from build123d import *

# Parameters (mm, degrees)
SCHIZZO1_W                   = 30
SCHIZZO1_H                   = 12
SCHIZZO1_R                   = 2.5
ESTRUSIONE_ESTRUSIONE1_DEPTH = 7.5
TAGLIO_ESTRUSIONE1_REACH     = 33.5
SCHIZZO3_R                   = 2.5


with BuildPart() as part:
    # Schizzo1 → Estrusione-Estrusione1 (new, symmetric)
    with BuildSketch(Plane.XY):
        Rectangle(SCHIZZO1_W, SCHIZZO1_H)
        Circle(SCHIZZO1_R, mode=Mode.SUBTRACT)
    extrude(amount=ESTRUSIONE_ESTRUSIONE1_DEPTH, both=True)

    # Taglio-Estrusione1: up to this face of the body (flat: up to its plane)
    taglio_estrusione1_end = Plane(part.part.faces().sort_by_distance((-15, 0, 0))[0])
    # Schizzo3 → Taglio-Estrusione1 (cut, up to the picked face)
    with BuildSketch(Plane(origin=(15, 0, 0), x_dir=(0, 0, -1), z_dir=(1, 0, 0)), mode=Mode.PRIVATE) as taglio_estrusione1_sk1:
        Circle(SCHIZZO3_R)
    taglio_estrusione1_tool1 = split(extrude(taglio_estrusione1_sk1.sketch, amount=-TAGLIO_ESTRUSIONE1_REACH, mode=Mode.PRIVATE), bisect_by=taglio_estrusione1_end, keep=Keep.BOTH, mode=Mode.PRIVATE)
    add(taglio_estrusione1_tool1.solids().sort_by(Axis((15, 0, 0), (-1, 0, 0)))[0], mode=Mode.SUBTRACT)


solid = part.part
Part model, mm, in its own coordinate system. Coordinates: 2 decimals unless noted, no trailing zeros. Loops run counter-clockwise (first coordinate to the right, second up) from the corner with the lowest first, then second, coordinate; pieces in that order, holes last. Notation, with made-up numbers: (-26, 4) -> (20, 4) arc R16 cw to (20, 9) -> close; hole circle Ø1 at (-27.75, 28). An arc over 180 degrees is marked (long way). Use a Markdown table: item, result. Add a question column.
Item 1: Band-saw the part on C-C on z = -3. Write the cut outline in (x, y).
Item 2: Flat gauge pin, fed straight in: P1, Ø6.5, axis at x = 0, y = 0, coming from the +Z side. Where does the tip first touch, or does it go through?
Item 3: Band-saw the part on A-A on y = 0. Write the cut outline in (x, z), plus the area to 3 significant figures.
Item 4: Probe probe 1 along Y at (x, z) = (1, 0); probe 2 along Z at (x, y) = (9.25, 0); probe 3 along X at (y, z) = (-0.25, -4). List the from-to ranges inside material, lowest first.
Item 5: Band-saw the part on D-D on x = -1. Write the cut outline in (y, z), plus the area to 3 significant figures.
Item 6: Pull direction X, two halves, no side cores. Call faces 1 (the cylindrical face through (-2.5, 0.1, -4.6)), 2 (the flat face through (0, 6, 0)), 3 (the flat face through (-15, 3, 0)), 4 (the cylindrical face through (-2.5, 0.1, 4.5)): +X half, -X half, draft (parallel to the pull), parting line (faces both ways), or undercut.
Item 7: Band-saw the part on B-B on z = 2. Write the cut outline in (x, y).
Geometry says:
| question | item | result |
|---|---|---|
| 1 | outline | (-15, -6) -> (15, -6) -> (15, 6) -> (-15, 6) -> close; hole circle Ø5 at (0, 0) |
| 2 | P1 | z = 7.5 |
| 3 | outline | (-15, -7.5) -> (-2.5, -7.5) -> (-2.5, -2.5) -> (-15, -2.5) -> close; (-15, 2.5) -> (-2.5, 2.5) -> (-2.5, 7.5) -> (-15, 7.5) -> close; (2.5, -7.5) -> (15, -7.5) -> (15, -2.5) -> (2.5, -2.5) -> close; (2.5, 2.5) -> (15, 2.5) -> (15, 7.5) -> (2.5, 7.5) -> close |
| 3 | area | 250 mm² |
| 4 | probe 1 | -6 to -2.5, 2.5 to 6 |
| 4 | probe 2 | -7.5 to -2.5, 2.5 to 7.5 |
| 4 | probe 3 | -15 to -2.49, 2.49 to 15 |
| 5 | outline | (-6, -7.5) -> (-2.29, -7.5) -> (-2.29, -1) arc R2.5 cw to (-2.29, 1) -> (-2.29, 7.5) -> (-6, 7.5) -> close; (2.29, -7.5) -> (6, -7.5) -> (6, 7.5) -> (2.29, 7.5) -> (2.29, 1) arc R2.5 cw to (2.29, -1) -> close |
| 5 | area | 111 mm² |
| 6 | face 1 | undercut |
| 6 | face 2 | draft |
| 6 | face 3 | -X half |
| 6 | face 4 | undercut |
| 7 | outline | (-15, -6) -> (15, -6) -> (15, -1.5) -> (2, -1.5) arc R2.5 cw to (-2, -1.5) -> (-15, -1.5) -> close; (-15, 1.5) -> (-2, 1.5) arc R2.5 cw to (2, 1.5) -> (15, 1.5) -> (15, 6) -> (-15, 6) -> close |
